Source: CAD feature listing. Evaluate the final solid. Frame: model axes, mm. Face numbers are marked on the shaded views. Give positions to 0.01 mm unless a question says otherwise; leave off trailing zeros. Write each loop counter-clockwise with the first axis right and the second up, starting at its lowest first coordinate (ties: lowest second). Pieces come first, ordered by that corner, then holes. Notation, with made-up numbers: (69.5, -34.5) -> (111.5, -34.5) arc R8 ccw to (111.5, -20.5) -> close; hole circle Ø8 at (57, 43). An arc over 180 degrees is marked (long way). Answer as a JSON object with one key per item and string values. Group by question number.
Item 1: Pull-direction query (X, two-part tool) for the marked faces 1, 2, 3 and 4; classes: pulls with the +X half, pulls with the -X half, needs draft (parallel to the pull), parting line crosses it, or undercut.
Item 2: First-contact query: pin 1 Ø7 at (x, y) = (20, -8) entering from -Z; pin 2 Ø4.5 at (x, y) = (-20, -8) entering from +Z. Flat tips, straight axial feed; report the tip coordinate or a pass-through.
Item 3: Section query C-C on x = 20. Return the cut outline in (y, z), plus the area to 3 significant figures.
Item 4: Section query B-B on z = -9. Return the cut outline in (x, y).
Item 5: Section query A-A on y = -8. Return the cut outline in (x, z) (3 decimals).
Item 6: Ray query, probe 1 along Y at (x, z) = (-20, -5.5); probe 2 along X at (y, z) = (-7.25, -3) (3 decimals); probe 3 along X at (y, z) = (-10.25, -11.5). Return the intervals inside material, ascending. Write a range as from..to.
Item 7: Section query D-D on y = -12. Return the cut outline in (x, z) (3 decimals), plus the area to 3 significant figures.
from build123d import *

# Parameters (mm, degrees)
F1_DEPTH = 16
F3_DEPTH = 12.501
F4_SIZE  = 1
F5_R     = 2


with BuildPart() as f1:
    # F0 (on Front) → F1 (new body)
    with BuildSketch(Plane.XZ):
        with BuildLine():
            Line((-6.375, 0), (-27, 0))
            Line((-27, 0), (-27, -12.5))
            Line((-27, -12.5), (27, -12.5))
            Line((27, -12.5), (27, 0))
            Line((27, 0), (6.375, 0))
            ThreePointArc((6.375, 0), (0, -6.375), (-6.375, 0))
        make_face()
    extrude(amount=F1_DEPTH)

    # F2 (on face) → F3 (cut, through all)
    with BuildSketch(Plane(origin=(0, 0, -12.5), x_dir=(1, 0, 0), z_dir=(0, 0, -1))):
        with BuildLine():
            Line((-22.75, 8), (-17.25, 8))
            ThreePointArc((-17.25, 8), (-20, 10.75), (-22.75, 8))
        make_face()
        with BuildLine():
            ThreePointArc((-22.75, 8), (-20, 5.25), (-17.25, 8))
            Line((-17.25, 8), (-22.75, 8))
        make_face()
        with BuildLine():
            ThreePointArc((22.75, 8), (20, 10.75), (17.25, 8))
            Line((17.25, 8), (22.75, 8))
        make_face()
        with BuildLine():
            Line((22.75, 8), (17.25, 8))
            ThreePointArc((17.25, 8), (20, 5.25), (22.75, 8))
        make_face()
    extrude(amount=-F3_DEPTH, mode=Mode.SUBTRACT)

    # F4
    f4_edges = [f1.edges().sort_by_distance(p)[0] for p in [
        (0, -16, -6.375),
        (0, 0, -6.375),
    ]]
    chamfer(f4_edges, length=F4_SIZE)

    # F5
    f5_edges = [f1.edges().sort_by_distance(p)[0] for p in [
        (-27, -16, -6.25),
        (27, -16, -6.25),
        (27, 0, -6.25),
        (-27, 0, -6.25),
    ]]
    fillet(f5_edges, radius=F5_R)


solid = f1.part
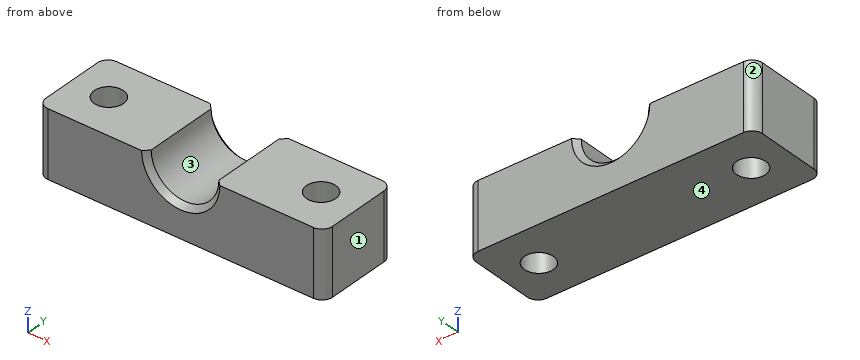
Worked answers:
{
 "1": {"face 1": "pulls with the +X half", "face 2": "pulls with the -X half", "face 3": "undercut", "face 4": "needs draft"},
 "2": {"pin 1": "z = -12.5", "pin 2": "through"},
 "3": {"outline": "(-16, -12.5) -> (-10.75, -12.5) -> (-10.75, 0) -> (-16, 0) -> close; (-5.25, -12.5) -> (0, -12.5) -> (0, 0) -> (-5.25, 0) -> close", "area": "131 mm^2"},
 "4": {"outline": "(-27, -14) arc R2 ccw to (-25, -16) -> (25, -16) arc R2 ccw to (27, -14) -> (27, -2) arc R2 ccw to (25, 0) -> (-25, 0) arc R2 ccw to (-27, -2) -> close; hole circle Ø5.5 at (-20, -8); hole circle Ø5.5 at (20, -8)"},
 "5": {"outline": "(-27, -12.5) -> (-22.75, -12.5) -> (-22.75, 0) -> (-27, 0) -> close; (-17.25, -12.5) -> (17.25, -12.5) -> (17.25, 0) -> (6.375, 0) arc R6.375 cw to (-6.375, 0) -> (-17.25, 0) -> close; (22.75, -12.5) -> (27, -12.5) -> (27, 0) -> (22.75, 0) -> close"},
 "6": {"probe 1": "-16..-10.75, -5.25..0", "probe 2": "-27..-22.646, -17.354..-5.625, 5.625..17.354, 22.646..27", "probe 3": "-27..-21.58, -18.42..18.42, 21.58..27"},
 "7": {"outline": "(-27, -12.5) -> (27, -12.5) -> (27, 0) -> (6.375, 0) arc R6.375 cw to (-6.375, 0) -> (-27, 0) -> close", "area": "611 mm^2"}
}
